```python
from build123d import *

# Parameters (mm, degrees)
SKETCH1_W           = 68.58
SKETCH1_H           = 88.9
BOSS_EXTRUDE1_DEPTH = 22.86
SKETCH2_W           = 55.88
SKETCH2_H           = 76.2
CUT_EXTRUDE1_DEPTH  = 13.97
SKETCH6_W           = 6.35
SKETCH6_H           = 6.35
CUT_EXTRUDE3_DEPTH  = 5.08
SKETCH7_W           = 2.54
SKETCH7_H           = 2.54
CUT_EXTRUDE4_DEPTH  = 114.882961412
SKETCH5_R           = 4.7625
CUT_EXTRUDE5_DEPTH  = 114.144099714


with BuildPart() as part:
    # Sketch1 → Boss-Extrude1 (new body)
    with BuildSketch(Plane(origin=(0, 0, 0), x_dir=(1, 0, 0), z_dir=(0, 1, 0))):
        with Locations((34.29, 44.45)):
            Rectangle(SKETCH1_W, SKETCH1_H)
    extrude(amount=BOSS_EXTRUDE1_DEPTH)

    # Sketch2 → Cut-Extrude1 (cut)
    with BuildSketch(Plane(origin=(0, 22.86, 0), x_dir=(1, 0, 0), z_dir=(0, 1, 0))):
        with Locations((34.29, 44.45)):
            Rectangle(SKETCH2_W, SKETCH2_H)
    extrude(amount=-CUT_EXTRUDE1_DEPTH, mode=Mode.SUBTRACT)

    # Sketch6 → Cut-Extrude3 (cut)
    with BuildSketch(Plane(origin=(0, 8.89, 0), x_dir=(1, 0, 0), z_dir=(0, 1, 0))):
        with Locations((18.034, 33.782)):
            Rectangle(SKETCH6_W, SKETCH6_H)
        with Locations((18.034, 13.716)):
            Rectangle(SKETCH6_W, SKETCH6_H)
    extrude(amount=-CUT_EXTRUDE3_DEPTH, mode=Mode.SUBTRACT)

    # Sketch7 → Cut-Extrude4 (cut, through all)
    with BuildSketch(Plane(origin=(0, 3.81, 0), x_dir=(1, 0, 0), z_dir=(0, 1, 0))):
        with Locations((18.034, 33.782)):
            Rectangle(SKETCH7_W, SKETCH7_H)
        with Locations((18.034, 13.716)):
            Rectangle(SKETCH7_W, SKETCH7_H)
    extrude(amount=-CUT_EXTRUDE4_DEPTH, mode=Mode.SUBTRACT)

    # Sketch5 → Cut-Extrude5 (cut, through all)
    with BuildSketch(Plane(origin=(0, 8.89, 0), x_dir=(1, 0, 0), z_dir=(0, 1, 0))):
        with Locations(Location((34.29, 72.644, 0), (0, 0, 270))):
            Circle(SKETCH5_R)
    extrude(amount=-CUT_EXTRUDE5_DEPTH, mode=Mode.SUBTRACT)


solid = part.part
```
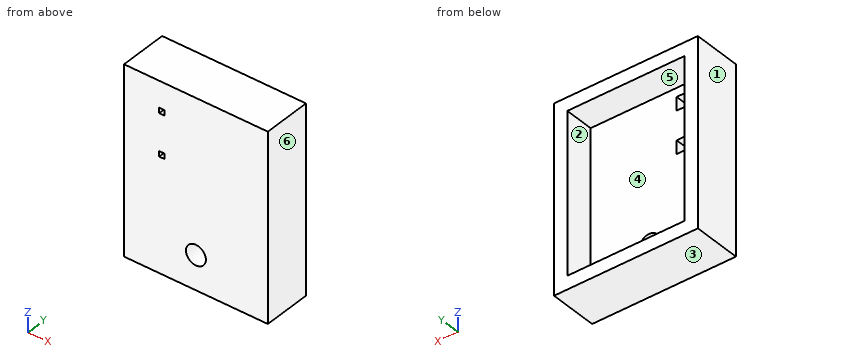
Geometry: final body of the model. Coordinates: model frame, mm. Face numbers are marked on the shaded views. A direction names the side the tool comes from. Coordinates: 2 decimals unless noted, no trailing zeros. Order: outer loops, then holes, each group sorted by start corner. A loop starts at its lowest first (then second) coordinate and runs counter-clockwise, first axis right, second up.
Item 1: Section query B-B (y = 6). Output: boundary loops of the cut face in (x, z) (1 decimal), then the cut area to 3 significant figures.
Answer:
outline: (0, -88.9) - (68.6, -88.9) - (68.6, 0) - (0, 0) - close; hole (14.9, -37) - (21.2, -37) - (21.2, -30.6) - (14.9, -30.6) - close; hole (14.9, -16.9) - (21.2, -16.9) - (21.2, -10.5) - (14.9, -10.5) - close; hole circle Ø9.5 at (34.3, -72.6)
area: 5,940 mm2
Item 2: Section query C-C (y = 16.5). Output: boundary loops of the cut face in (x, z).
Answer:
outline: (0, -88.9) - (68.58, -88.9) - (68.58, 0) - (0, 0) - close; hole (6.35, -82.55) - (62.23, -82.55) - (62.23, -6.35) - (6.35, -6.35) - close
Item 3: Section query A-A (x = 34.29). Output: boundary loops of the cut face in (y, z), then the cut area to 3 significant figures.
Answer:
outline: (0, -88.9) - (22.86, -88.9) - (22.86, -82.55) - (8.89, -82.55) - (8.89, -77.41) - (0, -77.41) - close; (0, -67.88) - (8.89, -67.88) - (8.89, -6.35) - (22.86, -6.35) - (22.86, 0) - (0, 0) - close
area: 883 mm2
Item 4: Draft query along X for the marked faces 3, 4, 5 and 6. Return one class per face: released by +X, released by -X, zero draft, split by the parting line, or undercut.
Answer:
face 3: zero draft
face 4: undercut
face 5: undercut
face 6: released by +X
Item 5: Material intervals for line 1 along Z through (x, y) = (16.5, 5.75); line 2 along Z through (x, y) = (57, 21.75); line 3 along X through (y, z) = (11.5, -56), sorted ascending.
Answer:
line 1: z = -88.9 to -36.96, -30.61 to -16.89, -10.54 to 0
line 2: z = -88.9 to -82.55, -6.35 to 0
line 3: x = 0 to 6.35, 62.23 to 68.58
Item 6: Contact query for flat-ended pins moving along their axis: P1, Ø12.5, axis at x = 34.29, z = -72.644, coming from the +Y side; P2, Ø1.5, axis at y = 6.5, z = -12, coming from the -X side. Output: stop coordinate, or through.
Answer:
P1: stops at y = 8.89
P2: stops at x = 0
Item 7: Section query D-D (z = -63). Output: boundary loops of the cut face in (x, y).
Answer:
outline: (0, 0) - (68.58, 0) - (68.58, 22.86) - (62.23, 22.86) - (62.23, 8.89) - (6.35, 8.89) - (6.35, 22.86) - (0, 22.86) - close
Item 8: Access query for the marked faces 1 and 2. Directions: +Z, -Z, +X, -X, +Y, -Y. A direction counts if a zero-diameter tool reaches every point of the face in a straight line with its end or side. Return the directions, or none.
Answer:
face 1: +Z, -Z, -X, +Y, -Y
face 2: +Y
